Can you work these out from the model? Positions are in its coordinate system, mm. A direction names the side the tool comes from. Round coordinates to 2 decimals unless told otherwise and drop trailing zeros. Write each loop counter-clockwise with the first axis right and the second up, starting at its lowest first coordinate (ties: lowest second). Pieces come first, ordered by that corner, then holes.
Q1. If we section it at C-C (y = 0.8): Please give me the cut outline in (x, z) (1 decimal).
Q2. Please list where these lines run through material, in increasing order: line 1 along Z through (x, y) = (9, 1.2); line 2 along X through (y, z) = (0.25, -5); line 3 along Z through (x, y) = (1, 0.75).
Q3. For faces 1 (the flat face through (8.6, 1.57, -2.67)), 2 (the flat face through (-4, 3.175, -3)), which set-ups out of +Z, -Z, +X, -X, +Y, -Y let a thin tool reach every point of the face, with its end or its side?
Q4. I'm going to push flat-ended pins straight in: pin 1 Ø1.5 at (x, y) = (-13.5, 2.5) entering from -Z; pin 2 Ø1 at (x, y) = (10, 0.5) entering from -Z; pin 3 Ø1.7 at (x, z) = (-22.48, -2.42) entering from +Y. Where does each tip first touch, or does it pass through?
Q5. If we section it at D-D (z = -14): Please give me the cut outline in (x, y) (3 decimals).
Q6. We'd pull the mould along X, two halves only. Please class faces 3 (the cylindrical face through (3.433, 1.565, 21.081)), 4 (the cylindrical face through (-25.56, 1.57, -2.45)), 5 (the cylindrical face through (2.611, 1.565, -30.638)): +X half, -X half, draft (parallel to the pull), parting line (faces both ways), or undercut.
Q7. If we section it at B-B (z = 8.5): Please give me the cut outline in (x, y) (3 decimals), plus the area to 3 significant figures.
Q8. If we section it at A-A (x = -2): Please give me the cut outline in (y, z) (3 decimals).
from build123d import *

# Parameters (mm, degrees)
SKETCH1_R           = 0.9525
BOSS_EXTRUDE1_DEPTH = 3.175


with BuildPart() as part:
    # Sketch1 → Boss-Extrude1 (new body)
    with BuildSketch(Plane(origin=(0, 0, 0), x_dir=(1, 0, 0), z_dir=(0, 1, 0))):
        with BuildLine():
            Line((0.836079848, 29.914691197), (-24.916908158, 4.139124102))
            ThreePointArc((-24.916908158, 4.139124102), (-25.559946724, 2.427169764), (-24.804168658, 0.761911295))
            Line((-24.804168658, 0.761911295), (0.802012418, -24.922477694))
            ThreePointArc((0.802012418, -24.922477694), (2.548586816, -25.648126247), (4.296057395, -24.924638497))
            Line((4.296057395, -24.924638497), (29.933843676, 0.727916893))
            ThreePointArc((29.933843676, 0.727916893), (30.658077132, 2.414753754), (30.022424716, 4.136926421))
            Line((30.022424716, 4.136926421), (4.329842419, 29.912525833))
            ThreePointArc((4.329842419, 29.912525833), (2.583410169, 30.638116576), (0.836079848, 29.914691197))
        make_face()
        with Locations(Location((2.67042066, 27.595082687, 0), (0, 0, 270))):
            Circle(SKETCH1_R, mode=Mode.SUBTRACT)
        with Locations(Location((-22.478149371, 2.417496952, 0), (0, 0, 270))):
            Circle(SKETCH1_R, mode=Mode.SUBTRACT)
        with Locations(Location((0.935185954, -5.154528514, 0), (0, 0, 270))):
            Circle(SKETCH1_R, mode=Mode.SUBTRACT)
        with Locations(Location((9.48030204, 4.90951313, 0), (0, 0, 270))):
            Circle(SKETCH1_R, mode=Mode.SUBTRACT)
        with Locations(Location((2.63009313, -20.568546616, 0), (0, 0, 270))):
            Circle(SKETCH1_R, mode=Mode.SUBTRACT)
        with Locations(Location((27.74686367, 2.479102218, 0), (0, 0, 270))):
            Circle(SKETCH1_R, mode=Mode.SUBTRACT)
        Polygon((8.316988679, -9.340962636), (-3.236630252, 2.247942235), (2.899230919, 8.38767289), (14.452988692, -3.201371075), align=None, mode=Mode.SUBTRACT)
    extrude(amount=BOSS_EXTRUDE1_DEPTH)


solid = part.part
A:
1. outline: (-24.9, -4.1) - (0.8, -29.9) arc R2.5 ccw to (4.3, -29.9) - (30, -4.1) arc R2.5 ccw to (29.9, -0.7) - (4.3, 24.9) arc R2.5 ccw to (0.8, 24.9) - (-24.8, -0.8) arc R2.4 ccw to start; hole circle Ø1.9 at (-22.5, -2.4); hole (-3.2, -2.2) - (2.9, -8.4) - (14.5, 3.2) - (8.3, 9.3) - close; hole circle Ø1.9 at (0.9, 5.2); hole circle Ø1.9 at (2.7, -27.6); hole circle Ø1.9 at (2.6, 20.6); hole circle Ø1.9 at (9.5, -4.9); hole circle Ø1.9 at (27.7, -2.5)
2. line 1: z = -25.23 to -5.73, -4.09 to -2.27, 8.66 to 20.22
2. line 2: x = -24.06 to -0.49, 6.28 to 8.53, 10.43 to 29.16
2. line 3: z = -30.06 to -6.49, 2 to 4.2, 6.1 to 25.1
3. face 1: +Y, -Y
3. face 2: +Z, -Z, +X, -X, +Y
4. pin 1: stops at z = -16.32
4. pin 2: stops at z = -24.73
4. pin 3: passes through
5. outline: (-15.065, 0) - (20.191, 0) - (20.191, 3.175) - (-15.065, 3.175) - close
6. face 3: undercut
6. face 4: -X half
6. face 5: parting line
7. outline: (-15.57, 0) - (7.479, 0) - (7.479, 3.175) - (-15.57, 3.175) - close; (9.157, 0) - (20.711, 0) - (20.711, 3.175) - (9.157, 3.175) - close
7. area: 110 mm2
8. outline: (0, -27.076) - (3.175, -27.076) - (3.175, -3.485) - (0, -3.485) - close; (0, -1.008) - (3.175, -1.008) - (3.175, 22.112) - (0, 22.112) - close
